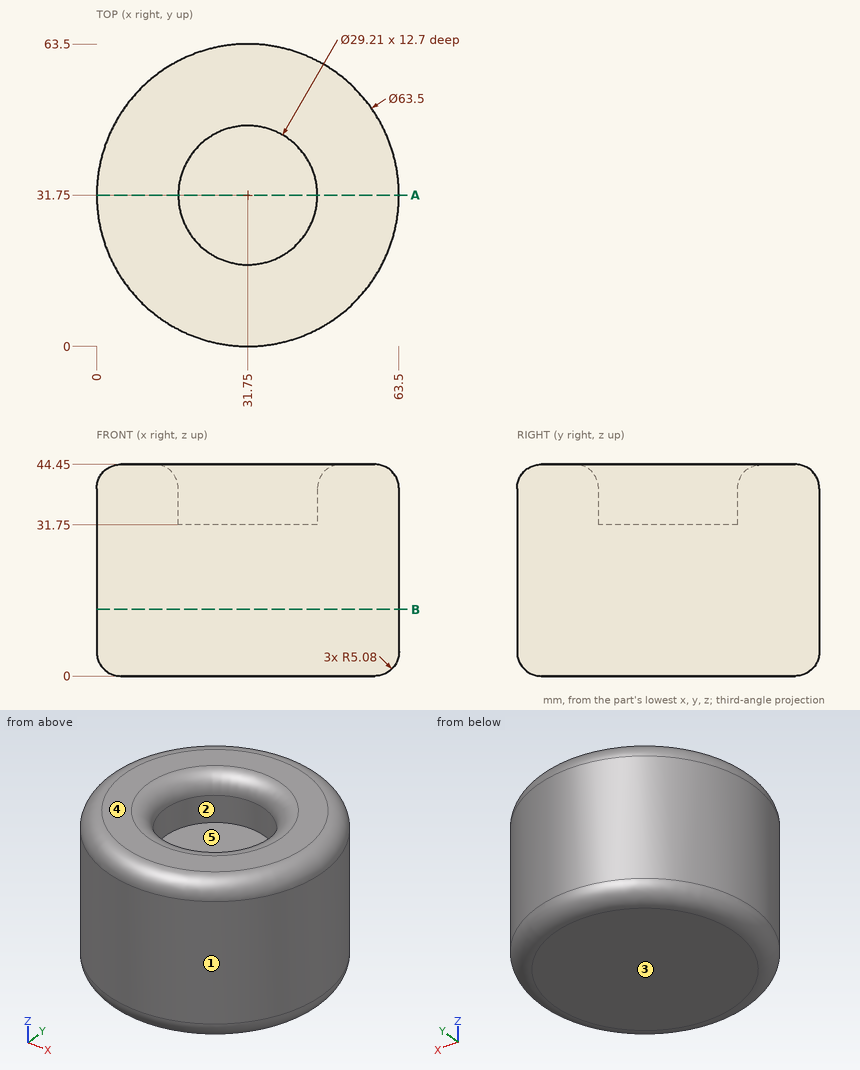
Verification items for this drawing (mm, ordinates from the low corner). A direction names the side the tool comes from. Coordinates: 2 decimals unless noted, no trailing zeros. Loops run counter-clockwise (first coordinate to the right, second up) from the corner with the lowest first, then second, coordinate; pieces in that order, holes last.
Item 1: Sectioned sample at A-A, the plane y = 31.75. Record the boundary of the cut face in (x, z) (3 decimals).
Item 2: Sectioned sample at B-B, the plane z = 14. Record the boundary of the cut face in (x, y).
Item 3: Thickness scan on line 1 (Y direction, x = 31, z = 36); line 2 (Y direction, x = 31.75, z = 37.75) (3 decimals); line 3 (X direction, y = 14.5, z = 26.5). Record the ranges inside material, lowest first.
Item 4: Access from +Z, -Z, +X, -X, +Y, -Y to the whole of each face (thin tool, end or side, straight path). Record for the marked faces 4 and 5.
Item 5: Go/stop test with flat-tipped pins: pin 1 Ø5 at (y, z) = (49.5, 24.5) entering from +X; pin 2 Ø14.5 at (x, y) = (26.5, 27.5) entering from +Z; pin 3 Ø1.5 at (x, z) = (36, 23.5) entering from +Y. Record where each tip stops, or that it passes through.
Item 6: Release check for a two-part mould opening along X. For the marked faces 1, 2 and 3 record: released by +X, released by -X, zero draft, split by the parting line, or undercut.
Check result:
1. outline: (0, 5.08) arc R5.08 ccw to (5.08, 0) - (58.42, 0) arc R5.08 ccw to (63.5, 5.08) - (63.5, 39.37) arc R5.08 ccw to (58.42, 44.45) - (51.435, 44.45) arc R5.08 ccw to (46.355, 39.37) - (46.355, 31.75) - (17.145, 31.75) - (17.145, 39.37) arc R5.08 ccw to (12.065, 44.45) - (5.08, 44.45) arc R5.08 ccw to (0, 39.37) - close
2. outline: circle Ø63.5 at (31.75, 31.75)
3. line 1: y = 0.01 to 17.16, 46.34 to 63.49
3. line 2: y = 0 to 17.145, 46.355 to 63.5
3. line 3: x = 5.09 to 58.41
4. face 4: +Z, +X, -X, +Y, -Y
4. face 5: +Z
5. pin 1: stops at x = 59.6
5. pin 2: stops at z = 31.75
5. pin 3: stops at y = 63.31
6. face 1: split by the parting line
6. face 2: undercut
6. face 3: zero draft
